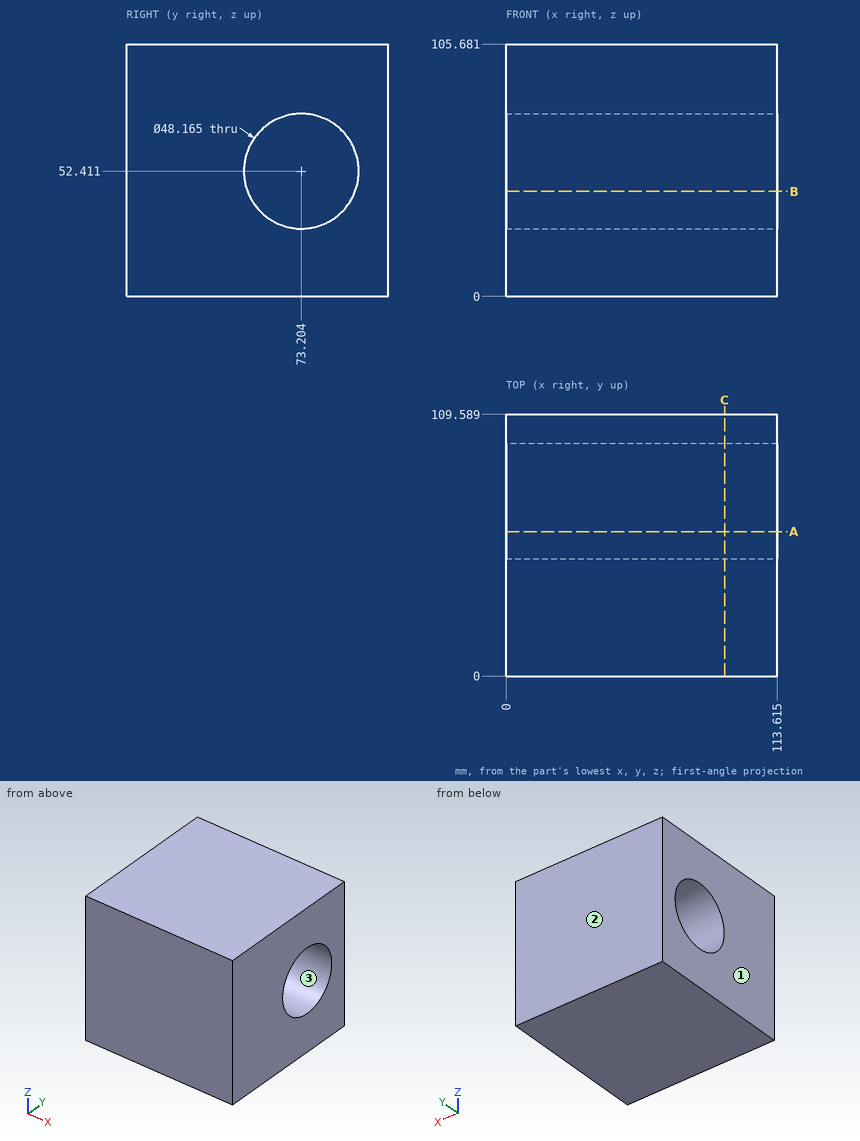
Source: three-view drawing plus pictorial views. Frame: mm from the lowest corner of the part. Coordinates: 2 decimals unless noted, no trailing zeros. Write each loop counter-clockwise with the first axis right and the second up, starting at its lowest first coordinate (ties: lowest second). Pieces come first, ordered by that corner, then holes. Notation, with made-up numbers: (26.25, -19.75) -> (53.25, -19.75) arc R29 cw to (53.25, 12.25) -> close; hole circle Ø2 at (54.25, -35.75). An arc over 180 degrees is marked (long way). Answer as a JSON object with one key per item and string values.
1. Section A-A on y = 60.5. Return the cut outline in (x, z) (1 decimal), then the cut area to 3 significant figures.
Result set:
{"outline": "(0, 0) -> (113.6, 0) -> (113.6, 32) -> (0, 32) -> close; (0, 72.9) -> (113.6, 72.9) -> (113.6, 105.7) -> (0, 105.7) -> close", "area": "7,360 mm2"}
2. Section B-B on z = 44. Return the cut outline in (x, y) (1 decimal), then the cut area to 3 significant figures.
Result set:
{"outline": "(0, 0) -> (113.6, 0) -> (113.6, 50.6) -> (0, 50.6) -> close; (0, 95.8) -> (113.6, 95.8) -> (113.6, 109.6) -> (0, 109.6) -> close", "area": "7,320 mm2"}
3. Mould query, pull axis Y, two halves, no side actions, for the marked faces 1, 2 and 3. Classes: released by +Y, released by -Y, zero draft, split by the parting line, or undercut.
Result set:
{"face 1": "zero draft", "face 2": "released by +Y", "face 3": "undercut"}
4. Material intervals for line 1 (Y direction, x = 54, z = 65.5); line 2 (Z direction, x = 47, y = 73); line 3 (Z direction, x = 75.5, y = 52.5) (1 decimal), sorted ascending. Write a range as from..to.
Result set:
{"line 1": "y = 0..52.99, 93.42..109.59", "line 2": "z = 0..28.33, 76.49..105.68", "line 3": "z = 0..40.1, 64.7..105.7"}
5. Section C-C on x = 91.5. Return the cut outline in (y, z) (1 decimal).
Result set:
{"outline": "(0, 0) -> (109.6, 0) -> (109.6, 105.7) -> (0, 105.7) -> close; hole circle Ø48.2 at (73.2, 52.4)"}
